```python
from build123d import *

# Parameters (mm, degrees)
ODGI_CIE_BAZOWE1_DEPTH     = 150
SZKIC8_W                   = 100
SZKIC8_H                   = 100
WYTNIJ_WYCI_GNI_CIE3_DEPTH = 10
ZAOKR_GLENIE3_R            = 30
ZAOKR_GLENIE4_R            = 30
OTW_R_POD_RUB_M51_D        = 5.5
OTW_R_POD_RUB_M51_DEPTH    = 14
OTW_R_POD_RUB_M51_TIP      = 1.652366702


# Sheet-metal steps are written as plain solids
with BuildPart() as part:
    # Szkic1 → Odgięcie bazowe1 (new body)
    with BuildSketch(Plane.XY):
        with BuildLine():
            Line((1038.6, -647.5), (1038.6, -624.284884098))
            ThreePointArc((1038.6, -624.284884098), (1038.264712868, -622.248777737), (1037.294258546, -620.427688781))
            Line((1037.294258546, -620.427688781), (963.094449397, -523.392669649))
            Line((963.094449397, -523.392669649), (964.683192246, -522.177804982))
            Line((964.683192246, -522.177804982), (1038.883001396, -619.212824114))
            ThreePointArc((1038.883001396, -619.212824114), (1040.159110622, -621.607484395), (1040.6, -624.284884098))
            Line((1040.6, -624.284884098), (1040.6, -647.5))
            Line((1040.6, -647.5), (1038.6, -647.5))
        make_face()
    extrude(amount=ODGI_CIE_BAZOWE1_DEPTH)

    # Szkic8 → Wytnij-wyciągnięcie3 (cut)
    with BuildSketch(Plane(origin=(355.1865636, 271.600659919, 0), x_dir=(0, 0, 1), z_dir=(-0.7943714246171976, -0.607432333475626, 0))):
        with Locations((75, -1050.782889378)):
            Rectangle(SZKIC8_W, SZKIC8_H)
    extrude(amount=-WYTNIJ_WYCI_GNI_CIE3_DEPTH, mode=Mode.SUBTRACT)

    # Zaokrąglenie3
    zaokr_glenie3_edges = [part.edges().sort_by_distance(p)[0] for p in [
        (1024.632054169, -602.222379777, 125),
    ]]
    fillet(zaokr_glenie3_edges, radius=ZAOKR_GLENIE3_R)

    # Zaokrąglenie4
    zaokr_glenie4_edges = [part.edges().sort_by_distance(p)[0] for p in [
        (1024.632054169, -602.222379777, 25),
    ]]
    fillet(zaokr_glenie4_edges, radius=ZAOKR_GLENIE4_R)

    # Otwór pod śrubę M51
    with Locations(Plane(origin=(1040.6, 0, 0), x_dir=(0, 0, -1), z_dir=(1, 0, 0))):
        with Locations((-30, -635.892442049), (-120, -635.892442049)):
            Hole(OTW_R_POD_RUB_M51_D / 2, depth=OTW_R_POD_RUB_M51_DEPTH)
            with Locations((0, 0, -(OTW_R_POD_RUB_M51_DEPTH + OTW_R_POD_RUB_M51_TIP / 2))):  # 118° drill point
                Cone(0, OTW_R_POD_RUB_M51_D / 2, OTW_R_POD_RUB_M51_TIP, mode=Mode.SUBTRACT)


solid = part.part
```
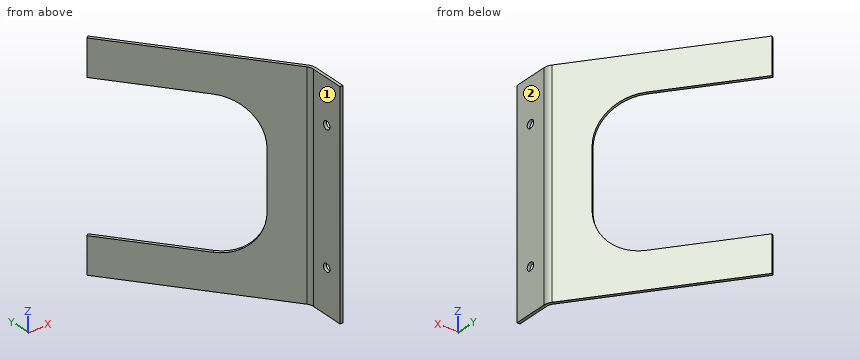
The model under review builds one solid part; all positions refer to its coordinate system, in mm. Face numbers are marked on the shaded views. A direction names the side the tool comes from. Coordinates: 2 decimals unless noted, no trailing zeros. Write each loop counter-clockwise with the first axis right and the second up, starting at its lowest first coordinate (ties: lowest second). Pieces come first, ordered by that corner, then holes. Notation, with made-up numbers: (34, 12.25) - (58, 12.25) arc R24 cw to (58, 31.25) - close; hole circle Ø1 at (19.25, 64). An arc over 180 degrees is marked (long way). Answer in a Markdown table with one row per item. Add a question column.
Q1. To check wall thickness, follow line 1 along Y through (x, z) = (1039.65, 120); line 2 along X through (y, z) = (-625.5, 107); line 3 along Y through (x, z) = (1039, 30). State the ranges of each line that lie inside material, in increasing order. Write a range as from..to.
Q2. Consider section A-A on z = 120. Give the boundary of the cut face in (x, y).
Q3. Consider section B-B on y = -544. Give the boundary of the cut face in (x, z), then the cut area to 3 significant figures.
Q4. Clearance check with flat-ended pins moving along their axes: pin 1 (7 mm diameter, centred on y = -633, z = 65, fed in from -X); pin 2 (1 mm diameter, centred on y = -622.5, z = 120.5, fed in from +X). State where each tip first meets the part, or that it passes through.
Q5. For the marked faces 1 and 2, list the 3-axis set-ups (+Z, -Z, +X, -X, +Y, -Y) from which the entire face can be reached by the end or side of a thin tool; tool diameter is ignored.
Answers below:
| question | item | result |
|---|---|---|
| 1 | line 1 | -647.5..-638.64, -633.14..-620.42 |
| 1 | line 2 | 1038.6..1040.6 |
| 1 | line 3 | -647.5..-638.64, -633.14..-619.37 |
| 2 | outline | (1015.69, -592.17) - (1037.29, -620.43) arc R6.35 cw to (1038.6, -624.28) - (1038.6, -633.14) - (1040.6, -633.14) - (1040.6, -624.28) arc R8.35 ccw to (1038.88, -619.21) - (1017.28, -590.96) - close; (1038.6, -647.5) - (1040.6, -647.5) - (1040.6, -638.64) - (1038.6, -638.64) - close |
| 3 | outline | (978.85, 0) - (981.37, 0) - (981.37, 25) - (978.85, 25) - close; (978.85, 125) - (981.37, 125) - (981.37, 150) - (978.85, 150) - close |
| 3 | area | 126 mm² |
| 4 | pin 1 | x = 1038.6 |
| 4 | pin 2 | x = 1040.5 |
| 5 | face 1 | +Z, -Z, -X, -Y |
| 5 | face 2 | +Z, -Z, +X, +Y, -Y |
